CAD build for the part. Positions are in the model's coordinates, mm. Round coordinates to 2 decimals unless told otherwise and drop trailing zeros. Loops run counter-clockwise (first coordinate to the right, second up) from the corner with the lowest first, then second, coordinate; pieces in that order, holes last. Notation, with made-up numbers: (34, 10.5) - (42, 10.5) arc R5 cw to (42, 19.5) - close; hole circle Ø2 at (15.5, 54.25). An arc over 180 degrees is marked (long way). Use one line per item in the form item = value.
from build123d import *

# Parameters (mm, degrees)
F1_DEPTH = 38.1


with BuildPart() as f1:
    # F0 (on Front) → F1 (new body)
    with BuildSketch(Plane.XZ):
        with BuildLine():
            Line((0, 17.304276), (0, 0))
            Line((0, 0), (25.4, 0))
            Line((25.4, 0), (25.4, 6.35))
            ThreePointArc((25.4, 6.35), (11.569272, 9.205286), (0, 17.304276))
        make_face()
        with BuildLine():
            Line((25.4, 6.35), (25.4, 0))
            Line((25.4, 0), (50.8, 0))
            Line((50.8, 0), (50.8, 17.304276))
            ThreePointArc((50.8, 17.304276), (39.230728, 9.205286), (25.4, 6.35))
        make_face()
    extrude(amount=F1_DEPTH)


solid = f1.part
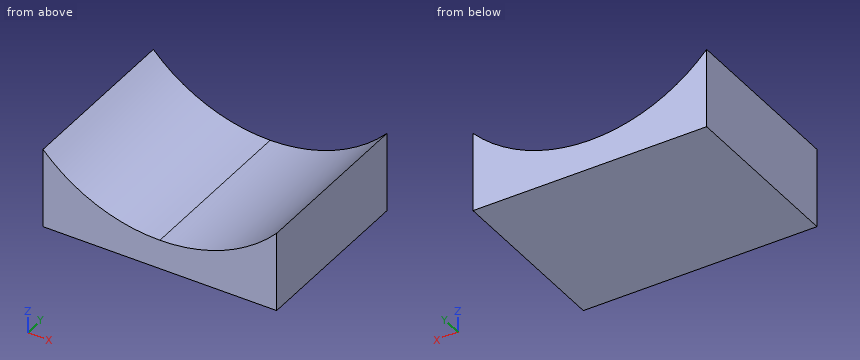
1) Slice it at B-B (y = -17). Write the cut outline in (x, z) (3 decimals).
Report:
outline = (0, 0) - (50.8, 0) - (50.8, 17.304) arc R34.925 cw to (25.4, 6.35) arc R34.925 cw to (0, 17.304) - close
2) Slice it at C-C (z = 13.75). Write the cut outline in (x, y), plus the area to 3 significant figures.
Report:
outline = (0, -38.1) - (3.9, -38.1) - (3.9, 0) - (0, 0) - close; (46.9, -38.1) - (50.8, -38.1) - (50.8, 0) - (46.9, 0) - close
area = 297 mm^2
3) Slice it at A-A (z = 8). Write the cut outline in (x, y).
Report:
outline = (0, -38.1) - (14.79, -38.1) - (14.79, 0) - (0, 0) - close; (36.01, -38.1) - (50.8, -38.1) - (50.8, 0) - (36.01, 0) - close
4) Flat gauge pin, fed straight in: pin 1 (1 mm diameter, centred on x = 30.5, y = -10, fed in from +Z). Where does the tip first touch, or does it go through?
Report:
pin_1 = 6.8
5) Slice it at D-D (x = 42). Write the cut outline in (y, z).
Report:
outline = (-38.1, 0) - (0, 0) - (0, 10.55) - (-38.1, 10.55) - close
6) Drill centre lines: probe 1 along X at (y, z) = (-22.5, 13.5); probe 2 along X at (y, z) = (-9, 16.25); probe 3 along Z at (x, y) = (26, -34). Where is each one in solid material? Low to high.
Report:
probe_1 = 0 to 4.23, 46.57 to 50.8
probe_2 = 0 to 1.04, 49.76 to 50.8
probe_3 = 0 to 6.36
